```python
from build123d import *

# Parameters (mm, degrees)
F0_R     = 1.8288
F0_W     = 123.19
F0_H     = 34.29
F1_DEPTH = 5.588
F2_R     = 4.445


with BuildPart() as f1:
    # F0 (on Right) → F1 (new body)
    with BuildSketch(Plane.YZ):
        with BuildLine():
            ThreePointArc((59, -22), (69.679492, 0), (59, 22))
            Line((59, 22), (-59, 22))
            ThreePointArc((-59, 22), (-69.679492, 0), (-59, -22))
            Line((-59, -22), (59, -22))
        make_face()
        with Locations((-65, -6.35)):
            Circle(F0_R, mode=Mode.SUBTRACT)
        with Locations((65, -6.35)):
            Circle(F0_R, mode=Mode.SUBTRACT)
        with Locations((-65, 0)):
            Circle(F0_R, mode=Mode.SUBTRACT)
        with Locations((-65, 6.35)):
            Circle(F0_R, mode=Mode.SUBTRACT)
        Rectangle(F0_W, F0_H, mode=Mode.SUBTRACT)
        with Locations((65, 0)):
            Circle(F0_R, mode=Mode.SUBTRACT)
        with Locations((65, 6.35)):
            Circle(F0_R, mode=Mode.SUBTRACT)
    extrude(amount=F1_DEPTH)

    # F2
    f2_edges = [f1.edges().sort_by_distance(p)[0] for p in [
        (2.794, -61.595, 17.145),
        (2.794, -61.595, -17.145),
        (2.794, 61.595, -17.145),
        (2.794, 61.595, 17.145),
    ]]
    fillet(f2_edges, radius=F2_R)


solid = f1.part
```
Source: CAD feature listing. Evaluate the final solid. Frame: model axes, mm. A direction names the side the tool comes from. Round coordinates to 2 decimals unless told otherwise and drop trailing zeros. Loops run counter-clockwise (first coordinate to the right, second up) from the corner with the lowest first, then second, coordinate; pieces in that order, holes last. Notation, with made-up numbers: M -23,-35 L 27,-35 A35 ccw 27,-1 Z; hole C 4,65 d9. An arc over 180 degrees is marked long. Put each result on its own line as item: value.
(1) Access query for faces 1 (the face through (5.588, -5, 18)), 2 (the face through (2.833, 60.258, -15.877)). Directions: +Z, -Z, +X, -X, +Y, -Y. A direction counts if a zero-diameter tool reaches every point of the face in a straight line with its end or side. Return the directions, or none.
Solutions:
face 1: +Z, -Z, +X, +Y, -Y
face 2: +X, -X
(2) Section B-B, the plane y = -48.5. Return loops of the section in (x, z) (3 decimals).
Solutions:
outline: M 0,-22 L 5.588,-22 L 5.588,-17.145 L 0,-17.145 Z; M 0,17.145 L 5.588,17.145 L 5.588,22 L 0,22 Z
(3) Ray query, line 1 (Z direction, x = 1.7, y = 0) (3 decimals); line 2 (Z direction, x = 1.9, y = 65); line 3 (Y direction, x = 3.95, z = -8) (3 decimals). Return the intervals inside material, ascending. Write a range as [from, to].
Solutions:
line 1: [-22, -17.145], [17.145, 22]
line 2: [-15.5, -8.18], [-4.52, -1.83], [1.83, 4.52], [8.18, 15.5]
line 3: [-68.512, -65.789], [-64.211, -61.595], [61.595, 64.211], [65.789, 68.512]
(4) Section C-C, the plane x = 3.7. State how many separate pieces and enclosed holes the cut face has, and give its area (3 significant figures).
Solutions:
separate pieces: 1
enclosed holes: 7
area: 1,580 mm²
(5) Section A-A, the plane z = 0. Return loops of the section in (x, y) (1 decimal), and give its area (3 significant figures).
Solutions:
outline: M 0,-69.7 L 5.6,-69.7 L 5.6,-66.8 L 0,-66.8 Z; M 0,-63.2 L 5.6,-63.2 L 5.6,-61.6 L 0,-61.6 Z; M 0,61.6 L 5.6,61.6 L 5.6,63.2 L 0,63.2 Z; M 0,66.8 L 5.6,66.8 L 5.6,69.7 L 0,69.7 Z
area: 49.5 mm²
(6) First-contact query: pin 1 (3 mm diameter, centred on y = 65, z = 6.35, fed in from -X); pin 2 (3 mm diameter, centred on x = 2.5, z = -1.5, fed in from +Y); pin 3 (4 mm diameter, centred on y = 65, z = 0, fed in from -X); pin 4 (3 mm diameter, centred on x = 2, z = -3, fed in from -Y). Flat tips, straight axial feed; report the tip coordinate or a pass-through.
Solutions:
pin 1: through
pin 2: y = 69.68
pin 3: x = 0
pin 4: y = -69.64
(7) Section D-D, the plane y = 65. Return loops of the section in (x, z).
Solutions:
outline: M 0,-15.5 L 5.59,-15.5 L 5.59,-8.18 L 0,-8.18 Z; M 0,-4.52 L 5.59,-4.52 L 5.59,-1.83 L 0,-1.83 Z; M 0,1.83 L 5.59,1.83 L 5.59,4.52 L 0,4.52 Z; M 0,8.18 L 5.59,8.18 L 5.59,15.5 L 0,15.5 Z
(8) Pull-direction query (Z, two-part tool) for faces 3 (the face through (2.755, -69.677, 0.354)), 4 (the face through (3, 1, 22)), 5 (the face through (2.755, 66.744, 0.549)), 6 (the face through (0, -5, 18)); classes: released by +Z, released by -Z, zero draft, split by the parting line, or undercut.
Solutions:
face 3: split by the parting line
face 4: released by +Z
face 5: undercut
face 6: zero draft
